Here's how the part is built. I have some questions about the finished solid (model axes, mm). Face numbers are marked on the shaded views. Round coordinates to 2 decimals unless told otherwise and drop trailing zeros. Order: outer loops, then holes, each group sorted by start corner. A loop starts at its lowest first (then second) coordinate and runs counter-clockwise, first axis right, second up. Notation, with made-up numbers: (35.25, 84) -> (78.25, 84) arc R17 cw to (78.25, 88) -> close; hole circle Ø4 at (-14, 6.25). An arc over 180 degrees is marked (long way). Use a Markdown table: item, result. Add a question column.
from build123d import *

# Parameters (mm, degrees)
FILLET1_R = 0.5


with BuildPart() as part:
    # Sketch1 → Revolve1 (revolve)
    with BuildSketch(Plane(origin=(0, 0, 0), x_dir=(1, 0, 0), z_dir=(0, 1, 0)), mode=Mode.PRIVATE) as revolve1_sk:
        Polygon((5, 0), (10, 0), (10, -2), (8.8, -2), (8.8, -10), (8.8, -21.398615454), (8.5, -23.1), (8.2, -23.1), (7.3, -10), (3.236730193, -10), align=None)
    revolve(revolve1_sk.sketch.rotate(Axis((0, 0, 0), (0, 0, 1)), 180), axis=Axis((0, 0, 0), (0, 0, 1)))  # turned: the seam where the file's is

    # Fillet1
    fillet1_edges = [part.edges().sort_by_distance(p)[0] for p in [
        (10, 0, 2),
        (10, 0, 0),
        (5, 0, 0),
    ]]
    fillet(fillet1_edges, radius=FILLET1_R)


solid = part.part
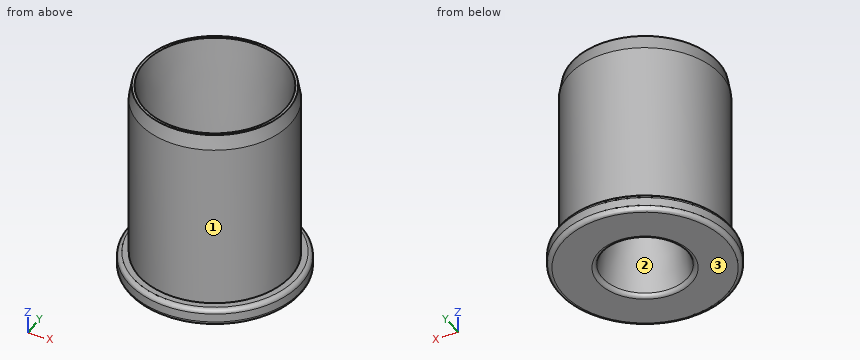
(1) I want a section at C-C on z = 18.75. List the corners of the cut face in (x, y) for me, and give its area (3 significant figures).
(2) Please list where these lines run through material, in increasing order: probe 1 along X at (y, z) = (7, 17.5); probe 2 along X at (y, z) = (0.5, 5.75); probe 3 along Y at (x, z) = (-0.25, 17.25). Write a range as from..to.
(3) I'm going to push flat-ended pins straight in: P1, Ø6, axis at x = 2.5, z = 11.5, coming from the +Y side; P2, Ø5, axis at x = -4, y = -2, coming from the +Z side; P3, Ø12, axis at y = 1.5, z = 19, coming from the +X side. Where does each tip first touch, or does it pass through?
(4) I want a section at A-A on y = 0. List the corners of the cut face in (x, z) for me.
(5) If we mould it in two halves opening along X, with no side actions, what happens to the marked faces 1, 2 and 3? For each: pulls with the +X half, pulls with the -X half, needs draft (parallel to the pull), parting line crosses it, or undercut.
(6) I want a section at D-D on z = 5. List the corners of the cut face in (x, y) for me.
Output:
| question | item | result |
|---|---|---|
| 1 | outline | circle Ø17.6 at (0, 0); hole circle Ø15.8 at (0, 0) |
| 1 | area | 47.2 mm² |
| 2 | probe 1 | -5.33..-3.48, 3.48..5.33 |
| 2 | probe 2 | -8.79..-3.95, 3.95..8.79 |
| 2 | probe 3 | -8.8..-7.79, 7.79..8.8 |
| 3 | P1 | y = 8.8 |
| 3 | P2 | z = 10 |
| 3 | P3 | x = 8.8 |
| 4 | outline | (-10, 0.5) arc R0.5 ccw to (-9.5, 0) -> (-5.42, 0) arc R0.5 ccw to (-4.93, 0.41) -> (-3.24, 10) -> (-7.3, 10) -> (-8.2, 23.1) -> (-8.5, 23.1) -> (-8.8, 21.4) -> (-8.8, 2) -> (-9.5, 2) arc R0.5 ccw to (-10, 1.5) -> close; (3.24, 10) -> (4.93, 0.41) arc R0.5 ccw to (5.42, 0) -> (9.5, 0) arc R0.5 ccw to (10, 0.5) -> (10, 1.5) arc R0.5 ccw to (9.5, 2) -> (8.8, 2) -> (8.8, 21.4) -> (8.5, 23.1) -> (8.2, 23.1) -> (7.3, 10) -> close |
| 5 | face 1 | parting line crosses it |
| 5 | face 2 | undercut |
| 5 | face 3 | needs draft |
| 6 | outline | circle Ø17.6 at (0, 0); hole circle Ø8.24 at (0, 0) |
